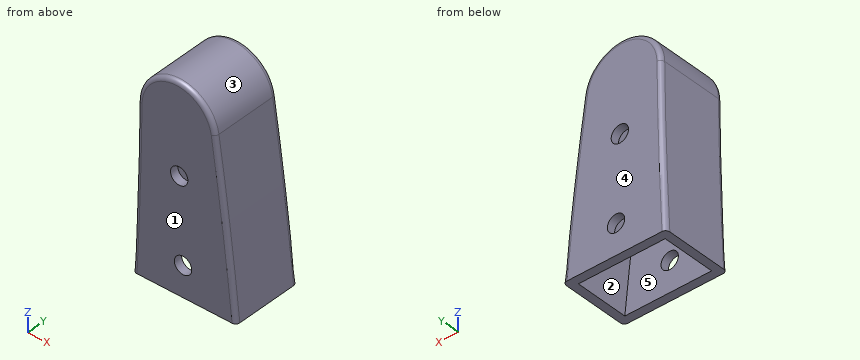
Autodesk Inventor part; units mm, degrees
ref_plane "YZ Plane" through (0, 0, 0) normal (1, 0, 0) x (0, 1, 0)
ref_plane "XZ Plane" through (0, 0, 0) normal (0, 1, 0) x (-1, 0, 0)
ref_plane "XY Plane" through (0, 0, 0) normal (0, 0, 1) x (1, 0, 0)
sketch "Sketch1" plane through (0, 0, 0) normal (0, 1, 0) x (-1, 0, 0)
  line L0 (0, 0) -> (-4, 0)
  line L1 (0, 0) -> (0, 36.6)
  line L2 (-24.4, 0) -> (-24.4, 6) construction
  line L3 (-18.4, 6) -> (-6, 6)
  line L4 (-6, 6) -> (-6, 30.6)
  line L5 (-6, 30.6) -> (-18.4, 30.6)
  line L6 (-18.4, 30.6) -> (-18.4, 6)
  line L7 (-24.4, 36.6) -> (-23.6295, 36.6) construction
  arc A0 (-20.163, 113.1038) -> (-23.4834, 116.9404) centre (-20, 116.6) ccw construction
  line L8 (-12.2, 4.1) -> (-12.2, 32.5) construction
  line L9 (-26.8761, 4.1) -> (8.0494, 4.1) construction
  line L10 (-27.3708, 32.5) -> (4.7796, 32.5) construction
  line L11 (-27.5308, 18.3) -> (1.4723, 18.3) construction
  arc A1 (-16.5002, 116.6381) -> (-9, 36.6) centre (470.9644, 121.9469) ccw construction
  line L12 (-23.6295, 36.6) -> (-13.0622, 36.6)
  line L13 (-9, 36.6) -> (0, 36.6)
  line L14 (-21.9951, 96.4905) -> (-19.8751, 96.6)
  line L15 (-19.8751, 96.6) -> (-15.8804, 96.8063) construction
  line L16 (-21.9951, 96.4905) -> (-25.9754, 96.8873) construction
  line L17 (-13.0622, 36.6) -> (-9.123, 37.2946) construction
  line L18 (-20, 116.6) -> (-16.5, 116.6) construction
  line L19 (-20, 116.6) -> (-20.7452, 100.6174) construction
  line L20 (-18.4, 6) -> (-24.4, 6)
  line L21 (-6, 6) -> (0, 6)
  arc A2 (-17.4, 0) -> (-14.7466, -6.9504) centre (-6.9703, 0) ccw
  arc A3 (-9.6573, 0) -> (-14.7466, -6.9504) centre (-0.5472, -12.0091) ccw
  arc A4 (-20.4, 0) -> (-13, -12) centre (-6.9703, 0) ccw
  arc A5 (-4, 0) -> (-13, -12) centre (1.9602, -13.8452) ccw
  line L22 (-14.7466, -6.9504) -> (-16.9833, -8.9496) construction
  line L23 (-14.7466, -6.9504) -> (-11.9734, -8.0949) construction
  line L24 (-20.4, 0) -> (-24.4, 0)
  line L25 (-17.4, 0) -> (-20.4, 0) construction
  line L26 (-9.6573, 0) -> (-17.4, 0)
  line L27 (-7.7289, -2.2981) -> (-9.6573, 0) construction
  arc A6 (-23.4834, 116.9404) -> (-20.163, 113.1038) centre (-20, 116.6) ccw construction
  line L28 (-21.4, -3.4679) -> (-21.4, 37.7463) construction
  line L29 (-24.4, 19.6) -> (-18.4, 19.6)
  line L30 (-6, 19.6) -> (0, 19.6)
  line L31 (-29.0378, 12.8) -> (2.5913, 12.8) construction
  arc A7 (-23.4618, 117.1157) -> (-24.4, 0) centre (391.9533, 55.2262) ccw construction
  arc A8 (-21.9951, 96.4905) -> (-23.6295, 36.6) centre (391.9533, 55.2262) ccw
  arc A9 (-19.8751, 96.6) -> (-13.0622, 36.6) centre (470.9644, 121.9469) ccw
  line L32 (-20.7452, 100.6174) -> (-20.9351, 96.5453) construction
  line L33 (-24.4, 6) -> (-24.4, 19.6)
  line L34 (-24.4, 19.6) -> (-24.4, 36.6) construction
  arc A10 (-15.3003, 116.6512) -> (-7.9935, 37.8) centre (470.9644, 121.9469) ccw
  line L35 (-7.9935, 37.8) -> (1.2, 37.8)
  line L36 (1.2, 37.8) -> (1.2, -1.2)
  line L37 (1.2, -1.2) -> (-3.7473, -1.2)
  arc A11 (-3.7473, -1.2) -> (-11.9132, -13.7694) centre (1.9602, -13.8452) ccw
  arc A12 (-21.5507, -1.2) -> (-11.9132, -13.7694) centre (-6.9703, 0) ccw
  line L38 (-21.5507, -1.2) -> (-25.45, -1.2)
  arc A13 (-24.6487, 117.2926) -> (-25.45, -1.2) centre (391.9533, 55.2262) ccw
  arc A14 (-15.3003, 116.6512) -> (-24.6487, 117.2926) centre (-20, 116.6) ccw
  line L39 (-15.8804, 96.8063) -> (-14.682, 96.8682)
  line L40 (-25.9754, 96.8873) -> (-27.1694, 97.0063)
  line L41 (-27.1694, 97.0063) -> (-14.682, 96.8682)
  point P0 (-20.2795, 110.6065)
  dimension "d4" = 6
  dimension "d5" = 24.6
  dimension "d6" = 12.4
  dimension "d7" = 6
  dimension "d15" = 7
  dimension "d17" = 9
  dimension "d21" = 20
  dimension "d23" = 80
  dimension "d24" = 20
  dimension "d29" = 170
  dimension "d30" = 6
  dimension "d31" = 10
  dimension "d43" = 4
  dimension "d44" = 3
  dimension "d45" = 4
  dimension "d50" = 13
  dimension "d51" = 12
  dimension "d52" = 130
  dimension "d89" = 6.8
  dimension "d90" = 28.4
  dimension "d107" = 420
  dimension "d108" = 4
  dimension "d109" = 4
  dimension "d114" = 1.2
  dimension "d115" = 1.2
extrude "Extrusion4" add sketch "Sketch1" along normal blind 8.4 contours A10 L41 A13 A14
shell "Shell1" thickness 1 removed faces 1 at (23.007, 2.8, 96.9603)
hole "Hole6" at (12.2, 0, 4.1) at (12.2, 0, 32.5) at (20.2795, 0, 110.6065) at (20.7452, 0, 100.6174) direction (0, 1, 0) diameter 2.1 end through all
fillet "Fillet12" radius 0.5 6 edges at (19.6783, 8.4, 121.289) (15.0918, 8.4, 106.7565) (26.0322, 8.4, 107.1647) (19.6783, 0, 121.289) (15.0918, 0, 106.7565) (26.0322, 0, 107.1647)
properties part number "LegEnd_Right_Head"
CAD build for the part. Positions are in the model's coordinates, mm. Face numbers are marked on the shaded views. A direction names the side the tool comes from. Round coordinates to 2 decimals unless told otherwise and drop trailing zeros. Order: outer loops, then holes, each group sorted by start corner. A loop starts at its lowest first (then second) coordinate and runs counter-clockwise, first axis right, second up.
Q1. Two-plate mould, pull along X, no slides. Class the marked faces 1, 2 and 3: pulls with the +X half, pulls with the -X half, needs draft (parallel to the pull), parting line crosses it, or undercut.
Q2. Wall check: L1, parallel to Y at x = 17, z = 113.75; L2, parallel to Z at x = 21, y = 0.5; L3, parallel to X at y = 4, z = 114.5. Give the ranges that are in metal, low to high.
Q3. Drop flat-ended pins along their axis: pin 1 (4 mm diameter, centred on y = 2, z = 118.5, fed in from -X); pin 2 (5 mm diameter, centred on y = 7, z = 113, fed in from +X); pin 3 (1 mm diameter, centred on y = 1.5, z = 114, fed in from +X). Give the stop position or say it passes through.
Q4. Which spindle directions (+Z, -Z, +X, -X, +Y, -Y) get a long thin tool onto all of the face, cutting with end or side? Do the marked faces 4 and 5. Say none if no direction does.
Q5. Slice it at A-A (y = 7). Write the cut outline in (x, z), and give its area (3 significant figures).
Results below:
1. face 1: needs draft
1. face 2: undercut
1. face 3: parting line crosses it
2. L1: y = 0 to 1, 7.4 to 8.4
2. L2: z = 96.94 to 99.6, 101.64 to 109.84, 111.37 to 121.19
2. L3: x = 15.27 to 16.27, 24.05 to 25.06
3. pin 1: stops at x = 15.3
3. pin 2: stops at x = 25.6
3. pin 3: stops at x = 25.2
4. face 4: +Z, -Z, +X, -X, +Y
4. face 5: -Z
5. outline: (14.68, 96.87) - (15.68, 96.88) arc R487.29 ccw to (16.3, 116.64) arc R3.7 cw to (23.66, 117.15) arc R420.2 cw to (26.17, 97) - (27.17, 97.01) arc R421.2 ccw to (24.65, 117.29) arc R4.7 ccw to (15.3, 116.65) arc R486.29 cw to start
5. area: 52.7 mm2
